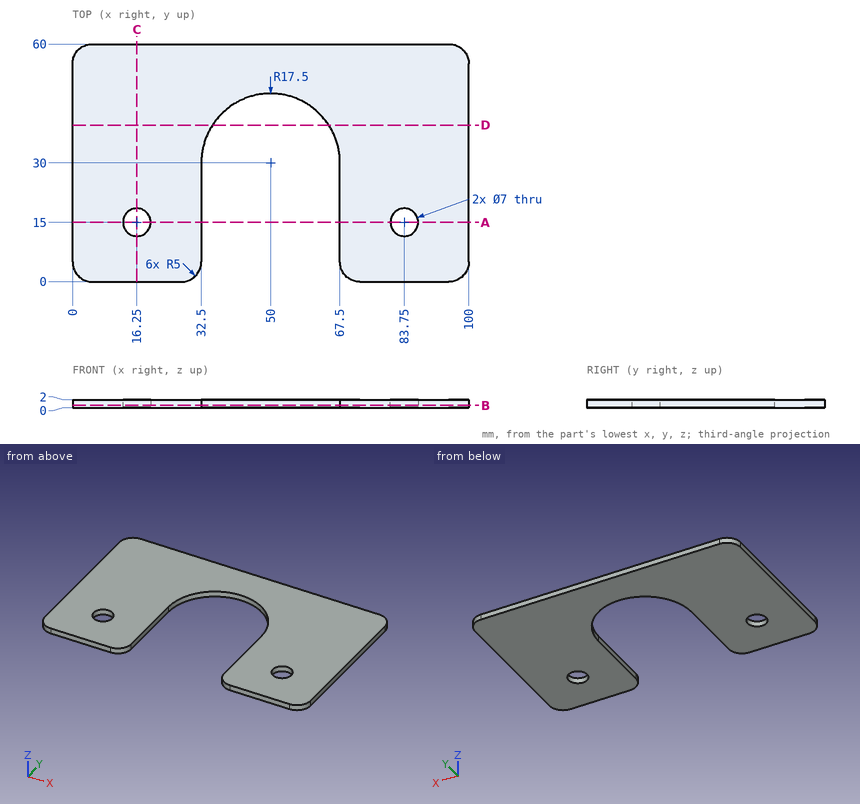
Input: dimensioned drawing with shaded views. Units: mm. Origin: part minimum x, y, z. Coordinates: 2 decimals unless noted, no trailing zeros. Order: outer loops, then holes, each group sorted by start corner. A loop starts at its lowest first (then second) coordinate and runs counter-clockwise, first axis right, second up.
1. Cut plane A-A, the plane y = 15. Return loops of the section in (x, z), plus the area to 3 significant figures.
Checked values:
outline: (0, 0) - (12.75, 0) - (12.75, 2) - (0, 2) - close; (19.75, 0) - (32.5, 0) - (32.5, 2) - (19.75, 2) - close; (67.5, 0) - (80.25, 0) - (80.25, 2) - (67.5, 2) - close; (87.25, 0) - (100, 0) - (100, 2) - (87.25, 2) - close
area: 102 mm2
2. Ray query, line 1 along Y through (x, z) = (16.25, 0.7); line 2 along X through (y, z) = (21.5, 1.8); line 3 along X through (y, z) = (3, 1.5). Return the intervals inside material, ascending.
Checked values:
line 1: y = 0 to 11.5, 18.5 to 60
line 2: x = 0 to 32.5, 67.5 to 100
line 3: x = 0.42 to 32.08, 67.92 to 99.58
3. Cut plane B-B, the plane z = 0.55. Return loops of the section in (x, y), plus the area to 3 significant figures.
Checked values:
outline: (0, 5) arc R5 ccw to (5, 0) - (27.5, 0) arc R5 ccw to (32.5, 5) - (32.5, 30) arc R17.5 cw to (67.5, 30) - (67.5, 5) arc R5 ccw to (72.5, 0) - (95, 0) arc R5 ccw to (100, 5) - (100, 55) arc R5 ccw to (95, 60) - (5, 60) arc R5 ccw to (0, 55) - close; hole circle Ø7 at (16.25, 15); hole circle Ø7 at (83.75, 15)
area: 4,360 mm2
4. Contact query for a flat-ended pin moving along its axis: P1, Ø4, axis at x = 83.75, y = 15, coming from the -Z side. Output: stop coordinate, or through.
Checked values:
P1: passes through
5. Cut plane C-C, the plane x = 16.25. Return loops of the section in (y, z), plus the area to 3 significant figures.
Checked values:
outline: (0, 0) - (11.5, 0) - (11.5, 2) - (0, 2) - close; (18.5, 0) - (60, 0) - (60, 2) - (18.5, 2) - close
area: 106 mm2
6. Cut plane D-D, the plane y = 39.5. Return loops of the section in (x, z).
Checked values:
outline: (0, 0) - (35.3, 0) - (35.3, 2) - (0, 2) - close; (64.7, 0) - (100, 0) - (100, 2) - (64.7, 2) - close
